Read the model definition and answer for the solid it produces. Units are mm, in the model's axes. Coordinates: 2 decimals unless noted, no trailing zeros. Loops run counter-clockwise (first coordinate to the right, second up) from the corner with the lowest first, then second, coordinate; pieces in that order, holes last. Notation, with made-up numbers: (23, 2.5) -> (72, 2.5) arc R16 cw to (72, 28.5) -> close; hole circle Ø11 at (58, 1). An arc over 180 degrees is marked (long way). Answer as a JSON object with one key per item and string values. Group by question number.
Q1. Determine the mould class of faces 1 (the cylindrical face through (-25.43, 10.65, 34.4)), 2 (the cylindrical face through (-12.82, 0.57, 0.6)), 3 (the cylindrical face through (-12.82, 1.59, 6.51)) for opening direction Z: released by +Z, released by -Z, zero draft, split by the parting line, or undercut.
Q2. The part is cut by section A-A on z = 27.5. Write down the section's boundary in (x, y).
Q3. This flat-tipped pin is pushed along its axis until it touches: P1, Ø3.5, axis at y = 3.5, z = 27.5, coming from the -X side. Where does it stop, or does it pass through?
Q4. The part is cut by section B-B on y = 3.5. Write down the section's boundary in (x, z).
Q5. The part is cut by section C-C on x = -12. Write down the section's boundary in (y, z), and give its area (3 significant figures).
Q6. Straight lines are drawn through the part: line 1 along Y through (x, z) = (-15.5, 7.5); line 2 along Z through (x, y) = (-18.75, 16.25); line 3 along Z through (x, y) = (-11, 3.75). For each, find the intervals that lie inside material, in ascending order. Write a range as [from, to].
from build123d import *

# Parameters (mm, degrees)
SKETCH_1_W          = 26
SKETCH_1_H          = 21
EXTRUDE_1_DEPTH     = 35
CUT_EXTRUDE_1_REACH = 50.394
SKETCH_2_R          = 2.15
FILLET_1_R          = 2


with BuildPart() as part:
    # 草图1 → 凸台-拉伸1 (new body)
    with BuildSketch(Plane.XY):
        with Locations((-13, 10.5)):
            Rectangle(SKETCH_1_W, SKETCH_1_H)
    extrude(amount=EXTRUDE_1_DEPTH)

    # 草图2 → 切除-拉伸1 (cut, up to next)
    with BuildSketch(Plane(origin=(0, 0, 0), x_dir=(0, 0, -1), z_dir=(1, 0, 0)), mode=Mode.PRIVATE) as cut_extrude_1_sk1:
        with Locations((-27.5, 17.5)):
            Circle(SKETCH_2_R)
    cut_extrude_1_tool1 = extrude(cut_extrude_1_sk1.sketch, amount=-CUT_EXTRUDE_1_REACH, mode=Mode.PRIVATE) & part.part
    # 草图2 → 切除-拉伸1 (cut, up to next)
    with BuildSketch(Plane(origin=(0, 0, 0), x_dir=(0, 0, -1), z_dir=(1, 0, 0)), mode=Mode.PRIVATE) as cut_extrude_1_sk2:
        with Locations((-27.5, 3.5)):
            Circle(SKETCH_2_R)
    cut_extrude_1_tool2 = extrude(cut_extrude_1_sk2.sketch, amount=-CUT_EXTRUDE_1_REACH, mode=Mode.PRIVATE) & part.part
    # 草图2 → 切除-拉伸1 (cut, up to next)
    with BuildSketch(Plane(origin=(0, 0, 0), x_dir=(0, 0, -1), z_dir=(1, 0, 0)), mode=Mode.PRIVATE) as cut_extrude_1_sk3:
        with Locations((-7.5, 17.5)):
            Circle(SKETCH_2_R)
    cut_extrude_1_tool3 = extrude(cut_extrude_1_sk3.sketch, amount=-CUT_EXTRUDE_1_REACH, mode=Mode.PRIVATE) & part.part
    # 草图2 → 切除-拉伸1 (cut, up to next)
    with BuildSketch(Plane(origin=(0, 0, 0), x_dir=(0, 0, -1), z_dir=(1, 0, 0)), mode=Mode.PRIVATE) as cut_extrude_1_sk4:
        with Locations((-7.5, 3.5)):
            Circle(SKETCH_2_R)
    cut_extrude_1_tool4 = extrude(cut_extrude_1_sk4.sketch, amount=-CUT_EXTRUDE_1_REACH, mode=Mode.PRIVATE) & part.part
    add(cut_extrude_1_tool1.solids().sort_by_distance((0, 17.5, 27.5))[0], mode=Mode.SUBTRACT)
    add(cut_extrude_1_tool2.solids().sort_by_distance((0, 3.5, 27.5))[0], mode=Mode.SUBTRACT)
    add(cut_extrude_1_tool3.solids().sort_by_distance((0, 17.5, 7.5))[0], mode=Mode.SUBTRACT)
    add(cut_extrude_1_tool4.solids().sort_by_distance((0, 3.5, 7.5))[0], mode=Mode.SUBTRACT)

    # 圆角1
    fillet_1_edges = [part.edges().sort_by_distance(p)[0] for p in [
        (-26, 10.5, 35),
        (-13, 0, 35),
        (0, 10.5, 35),
        (-13, 0, 0),
        (-26, 10.5, 0),
        (-13, 21, 0),
        (0, 10.5, 0),
        (-13, 21, 35),
    ]]
    fillet(fillet_1_edges, radius=FILLET_1_R)


solid = part.part
Final values:
{
 "1": {"face 1": "released by +Z", "face 2": "released by -Z", "face 3": "undercut"},
 "2": {"outline": "(-26, 0) -> (0, 0) -> (0, 1.35) -> (-26, 1.35) -> close; (-26, 5.65) -> (0, 5.65) -> (0, 15.35) -> (-26, 15.35) -> close; (-26, 19.65) -> (0, 19.65) -> (0, 21) -> (-26, 21) -> close"},
 "3": {"P1": "passes through"},
 "4": {"outline": "(-26, 2) arc R2 ccw to (-24, 0) -> (-2, 0) arc R2 ccw to (0, 2) -> (0, 5.35) -> (-26, 5.35) -> close; (-26, 9.65) -> (0, 9.65) -> (0, 25.35) -> (-26, 25.35) -> close; (-26, 29.65) -> (0, 29.65) -> (0, 33) arc R2 ccw to (-2, 35) -> (-24, 35) arc R2 ccw to (-26, 33) -> close"},
 "5": {"outline": "(0, 2) arc R2 ccw to (2, 0) -> (19, 0) arc R2 ccw to (21, 2) -> (21, 33) arc R2 ccw to (19, 35) -> (2, 35) arc R2 ccw to (0, 33) -> close; hole circle Ø4.3 at (3.5, 7.5); hole circle Ø4.3 at (3.5, 27.5); hole circle Ø4.3 at (17.5, 7.5); hole circle Ø4.3 at (17.5, 27.5)", "area": "673 mm2"},
 "6": {"line 1": "y = [0, 1.35], [5.65, 15.35], [19.65, 21]", "line 2": "z = [0, 5.75], [9.25, 25.75], [29.25, 35]", "line 3": "z = [0, 5.36], [9.64, 25.36], [29.64, 35]"}
}
